```python
from build123d import *

# Parameters (mm, degrees)
BOSS_EXTRUDE1_DEPTH = 20
FILLET3_R           = 5


with BuildPart() as part:
    # Sketch1 → Boss-Extrude1 (new, symmetric)
    with BuildSketch(Plane.XY):
        Polygon((0, 0), (0, 74), (2, 74), (20.281232104, 36.965983625), (5, 0), align=None)
    extrude(amount=BOSS_EXTRUDE1_DEPTH, both=True)

    # Fillet3
    # the kernel refuses this fillet: 5 mm, written as the material it takes off along each edge
    with BuildSketch(Plane(origin=(2, 74, 27.377711493), x_dir=(0.4426407168839213, -0.8966990552891692, 0), z_dir=(0, 0, -1))) as fillet3_piece_1:
        with BuildLine():
            CenterArc((2.951084597, 5), FILLET3_R, 219.89034736, 50.10965264)
            Line((-0.885281434, 1.793398111), (-0.962008754, 1.729266073))
            ThreePointArc((-0.962008754, 1.729266073), (-0.532310622, 0.852434984), (-0.089669906, -0.044264072))
            Line((-0.089669906, -0.044264072), (0, -0.1))
            Line((0, -0.1), (2.951084597, -0.1))
            Line((2.951084597, -0.1), (2.951084597, 0))
        make_face()
    extrude(amount=54.755422985, mode=Mode.SUBTRACT)


solid = part.part
```
Can you work these out from the model? Positions are in its coordinate system, mm. Give positions to 0.01 mm unless a question says otherwise; leave off trailing zeros. Loops run counter-clockwise (first coordinate to the right, second up) from the corner with the lowest first, then second, coordinate; pieces in that order, holes last. Notation, with made-up numbers: M -12,-39 L 13,-39 A31 cw 13,-12 Z; hole C 9,-13.5 d5. An arc over 180 degrees is marked long. One line per item, written item: value.
(1) Suppose I cut it at B-B on y = 33.5. List the corners of the cut face in (x, z) for me.
Returned:
outline: M 0,-20 L 18.85,-20 L 18.85,20 L 0,20 Z
(2) Suppose I cut it at A-A on z = 2. List the corners of the cut face in (x, y) for me, plus the area to 3 significant figures.
Returned:
outline: M 0,0 L 5,0 L 20.28,36.97 L 3.31,71.35 A5 ccw 0,74 Z
area: 879 mm^2
(3) Will these pins go through, and if not, where does the flat tip stop? pin 1 (8 mm diameter, centred on x = 16, z = -11, fed in from +Y); pin 2 (4 mm diameter, centred on y = 53, z = -1.5, fed in from +X).
Returned:
pin 1: y = 53.74
pin 2: x = 13.35
(4) Suppose I cut it at C-C on x = 8.25. List the corners of the cut face in (y, z) for me, plus the area to 3 significant figures.
Returned:
outline: M 7.86,-20 L 61.34,-20 L 61.34,20 L 7.86,20 Z
area: 2,140 mm^2
(5) I need wall thicknesses on line 1 (Y direction, x = 9, z = -11); line 2 (Y direction, x = 6, z = -8); line 3 (X direction, y = 16, z = 13). Which ranges of each line are inside material? Lowest first, please.
Returned:
line 1: 9.68 to 59.82
line 2: 2.42 to 65.9
line 3: 0 to 11.61
